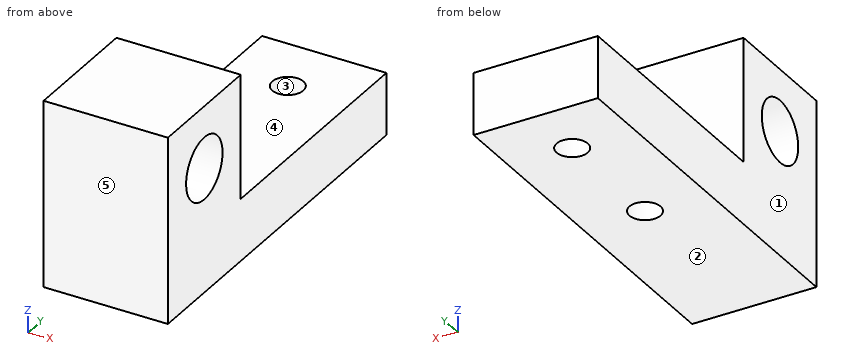
from build123d import *

# Parameters (mm, degrees)
F0_W     = 20
F0_H     = 60
F1_DEPTH = 10
F2_W     = 20
F2_H     = 20
F3_DEPTH = 20
F5_D     = 5
F7_D     = 5
F9_D     = 10


with BuildPart() as f1:
    # F0 (on Top) → F1 (new body)
    with BuildSketch(Plane.XY):
        Rectangle(F0_W, F0_H)
    extrude(amount=F1_DEPTH)

    # F2 (on face) → F3 (join)
    with BuildSketch(Plane.XY.offset(10)):
        with Locations((0, -20)):
            Rectangle(F2_W, F2_H)
    extrude(amount=F3_DEPTH)

    # F5 (through all)
    with Locations(Plane.XY.offset(10)):
        with Locations((0, 20)):
            Hole(F5_D / 2)

    # F7 (through all)
    with Locations(Plane.XY.offset(10)):
        with Locations((0, 0)):
            Hole(F7_D / 2)

    # F9 (through all)
    with Locations(Plane(origin=(-10, 0, 0), x_dir=(0, -1, 0), z_dir=(-1, 0, 0))):
        with Locations((20, 20)):
            Hole(F9_D / 2)


solid = f1.part
Can you work these out from the model? Positions are in its coordinate system, mm. Face numbers are marked on the shaded views. A direction names the side the tool comes from. Give positions to 0.01 mm unless a question says otherwise; leave off trailing zeros. Order: outer loops, then holes, each group sorted by start corner. A loop starts at its lowest first (then second) coordinate and runs counter-clockwise, first axis right, second up. Notation, with made-up numbers: (-13.5, 55.25) - (25.5, 55.25) arc R21 cw to (25.5, 91.25) - close; hole circle Ø4 at (84, 67). An arc over 180 degrees is marked (long way). Write each question's results on one line, items separated by ' | '.
1) If we mould it in two halves opening along X, with no side actions, what happens to the marked faces 1, 2 and 3? For each: pulls with the +X half, pulls with the -X half, needs draft (parallel to the pull), parting line crosses it, or undercut.
Final values:
face 1: pulls with the -X half | face 2: needs draft | face 3: undercut
2) Please list where these lines run through material, in increasing order: line 1 along Y through (x, z) = (0, 8); line 2 along Y through (x, z) = (-0.75, 6.75); line 3 along Z through (x, y) = (5.25, 17). Write a range as [from, to].
Final values:
line 1: y = [-30, -2.5], [2.5, 17.5], [22.5, 30] | line 2: y = [-30, -2.38], [2.38, 17.62], [22.38, 30] | line 3: z = [0, 10]
3) Suppose I cut it at A-A, the plane x = 0. Write out the boundary of the cut face in (y, z), then the cut area to 3 significant figures.
Final values:
outline: (-30, 0) - (-2.5, 0) - (-2.5, 10) - (-10, 10) - (-10, 30) - (-30, 30) - close; (2.5, 0) - (17.5, 0) - (17.5, 10) - (2.5, 10) - close; (22.5, 0) - (30, 0) - (30, 10) - (22.5, 10) - close; hole circle Ø10 at (-20, 20) | area: 821 mm^2
4) On a 3-axis mill with a long thin cutter (end or side, diameter ignored), from which of +Z, -Z, +X, -X, +Y, -Y can I reach the whole of each face in a straight line? I mean the marked faces 4 and 5. Say none if no direction works.
Final values:
face 4: +Z, +X, -X, +Y | face 5: +Z, -Z, +X, -X, -Y
5) Suppose I cut it at B-B, the plane y = -20. Write out the boundary of the cut face in (x, z), then the cut area to 3 significant figures.
Final values:
outline: (-10, 0) - (10, 0) - (10, 15) - (-10, 15) - close; (-10, 25) - (10, 25) - (10, 30) - (-10, 30) - close | area: 400 mm^2
6) I'm going to push flat-ended pins straight in: pin 1 Ø6 at (x, z) = (-1, 19.5) entering from +Y; pin 2 Ø8 at (x, y) = (0, 20) entering from +Z. Where does each tip first touch, or does it pass through?
Final values:
pin 1: stops at y = -10 | pin 2: stops at z = 10
7) Suppose I cut it at C-C, the plane z = 5.5. Write out the boundary of the cut face in (x, y), then the cut area to 3 significant figures.
Final values:
outline: (-10, -30) - (10, -30) - (10, 30) - (-10, 30) - close; hole circle Ø5 at (0, 0); hole circle Ø5 at (0, 20) | area: 1,160 mm^2
8) Suppose I cut it at D-D, the plane x = 4.5. Write out the boundary of the cut face in (y, z), then the cut area to 3 significant figures.
Final values:
outline: (-30, 0) - (30, 0) - (30, 10) - (-10, 10) - (-10, 30) - (-30, 30) - close; hole circle Ø10 at (-20, 20) | area: 921 mm^2
